Geometry check sheet. Reference: the model listing, model coordinates, mm. A direction names the side the tool comes from. Give positions to 0.01 mm unless a question says otherwise; leave off trailing zeros. Write each loop counter-clockwise with the first axis right and the second up, starting at its lowest first coordinate (ties: lowest second). Pieces come first, ordered by that corner, then holes. Notation, with made-up numbers: (-35.5, -11) -> (-4.5, -11) arc R17 ccw to (-4.5, 6) -> close; hole circle Ø5 at (33.5, 46.25). An arc over 180 degrees is marked (long way). One line per item, written item: value.
from build123d import *

# Parameters (mm, degrees)
BOSS_EXTRUDE1_DEPTH          = 3.175
SKETCH2_W                    = 2.75
SKETCH2_H                    = 2.5
SKETCH2_H_2                  = 4
SKETCH2_W_2                  = 1.125
SKETCH2_H_3                  = 7.5
CUT_EXTRUDE1_DEPTH           = 291.017379867
CIRPATTERN1_COUNT            = 4
F_3_0_3_DIAMETER_HOLE1_D     = 3
F_8_0_8_DIAMETER_HOLE1_D     = 8
F_8_0_8_DIAMETER_HOLE1_DEPTH = 6.35


with BuildPart() as part:
    # Sketch1 → Boss-Extrude1 (new, symmetric)
    with BuildSketch(Plane(origin=(0, 0, 0), x_dir=(1, 0, 0), z_dir=(0, 1, 0))):
        with BuildLine():
            Line((88.388347648, 98.994949366), (64.667874078, 75.274475795))
            ThreePointArc((64.667874078, 75.274475795), (-70.171862751, 70.171862751), (-75.274475795, -64.667874078))
            Line((-75.274475795, -64.667874078), (-98.994949366, -88.388347648))
            Line((-98.994949366, -88.388347648), (17.67766953, -205.060966544))
            Line((17.67766953, -205.060966544), (205.060966544, -17.67766953))
            Line((205.060966544, -17.67766953), (88.388347648, 98.994949366))
        make_face()
        with BuildLine():
            ThreePointArc((-64.667874078, -75.274475795), (0, -99.238), (64.667874078, -75.274475795))
            Line((64.667874078, -75.274475795), (95.45941546, -106.066017178))
            Line((95.45941546, -106.066017178), (17.67766953, -183.847763109))
            Line((17.67766953, -183.847763109), (-77.781745931, -88.388347648))
            Line((-77.781745931, -88.388347648), (-64.667874078, -75.274475795))
        make_face(mode=Mode.SUBTRACT)
        with BuildLine():
            ThreePointArc((75.274475795, -64.667874078), (99.238, 0), (75.274475795, 64.667874078))
            Line((75.274475795, 64.667874078), (88.388347648, 77.781745931))
            Line((88.388347648, 77.781745931), (183.847763109, -17.67766953))
            Line((183.847763109, -17.67766953), (106.066017178, -95.45941546))
            Line((106.066017178, -95.45941546), (75.274475795, -64.667874078))
        make_face(mode=Mode.SUBTRACT)
        with BuildLine():
            Line((-7.5, -7.5), (-7.5, -83.903460262))
            ThreePointArc((-7.5, -83.903460262), (-59.565261034, -59.565261034), (-83.903460262, -7.5))
            Line((-83.903460262, -7.5), (-7.5, -7.5))
        make_face(mode=Mode.SUBTRACT)
        with BuildLine():
            ThreePointArc((83.903460262, -7.5), (59.565261034, -59.565261034), (7.5, -83.903460262))
            Line((7.5, -83.903460262), (7.5, -7.5))
            Line((7.5, -7.5), (83.903460262, -7.5))
        make_face(mode=Mode.SUBTRACT)
        with BuildLine():
            Line((-7.5, 7.5), (-83.903460262, 7.5))
            ThreePointArc((-83.903460262, 7.5), (-59.565261034, 59.565261034), (-7.5, 83.903460262))
            Line((-7.5, 83.903460262), (-7.5, 7.5))
        make_face(mode=Mode.SUBTRACT)
        with BuildLine():
            ThreePointArc((7.5, 83.903460262), (59.565261034, 59.565261034), (83.903460262, 7.5))
            Line((83.903460262, 7.5), (7.5, 7.5))
            Line((7.5, 7.5), (7.5, 83.903460262))
        make_face(mode=Mode.SUBTRACT)
    extrude(amount=BOSS_EXTRUDE1_DEPTH, both=True)

    # Sketch2 → Cut-Extrude1 (cut, symmetric)
    with BuildSketch(Plane(origin=(0, 0, 0), x_dir=(1, 0, 0), z_dir=(0, 1, 0))):
        with Locations((0, 86.488)):
            Rectangle(SKETCH2_W, SKETCH2_H)
        with Locations((0, 89.738)):
            Rectangle(SKETCH2_W, SKETCH2_H_2)
        with Locations((1.9375, 89.738)):
            Rectangle(SKETCH2_W_2, SKETCH2_H_2)
        with Locations((0, 95.488)):
            Rectangle(SKETCH2_W, SKETCH2_H_3)
        with Locations((-1.9375, 89.738)):
            Rectangle(SKETCH2_W_2, SKETCH2_H_2)
    cut_extrude1 = extrude(amount=CUT_EXTRUDE1_DEPTH, both=True, mode=Mode.SUBTRACT)

    # CirPattern1: Cut-Extrude1 ×4 about axis
    cirpattern1_axis = Axis((0, 0, 0), (0, 1, 0))
    for i in range(1, CIRPATTERN1_COUNT):
        add(cut_extrude1.rotate(cirpattern1_axis, i * 360 / CIRPATTERN1_COUNT), mode=Mode.SUBTRACT)

    # Ø3.0 (3) Diameter Hole1 (through all)
    with Locations(Plane(origin=(0, 3.175, 0), x_dir=(1, 0, 0), z_dir=(0, 1, 0))):
        with Locations((-64.868561892, -64.868561892), (0, 0), (-64.868561892, 64.868561892), (64.868561892, 64.868561892), (64.868561892, -64.868561892)):
            Hole(F_3_0_3_DIAMETER_HOLE1_D / 2)

    # Ø8.0 (8) Diameter Hole1
    with Locations(Plane(origin=(0, 3.175, 0), x_dir=(1, 0, 0), z_dir=(0, 1, 0))):
        with Locations((0, 0)):
            Hole(F_8_0_8_DIAMETER_HOLE1_D / 2, depth=F_8_0_8_DIAMETER_HOLE1_DEPTH)


solid = part.part
1) Depth check by flat-ended pin: pin 1 Ø2 at (y, z) = (2.5, 69.5) entering from +X; pin 2 Ø2.5 at (x, z) = (64.87, 64.87) entering from -Y; pin 3 Ø1.5 at (x, y) = (-67.5, -2) entering from +Z; pin 4 Ø1 at (x, y) = (59.5, -2) entering from +Z. Enter the tip coordinate at first touch or a pass-through.
Verdict:
pin 1: x = 154.24
pin 2: through
pin 3: z = 120.63
pin 4: z = 163.74
2) Sectioned sample at A-A on x = -15. Record the cut outline in (y, z) (3 decimals).
Verdict:
outline: (-3.175, -98.098) -> (3.175, -98.098) -> (3.175, -82.892) -> (-3.175, -82.892) -> close; (-3.175, -7.5) -> (3.175, -7.5) -> (3.175, 7.5) -> (-3.175, 7.5) -> close; (-3.175, 82.892) -> (3.175, 82.892) -> (3.175, 98.098) -> (-3.175, 98.098) -> close; (-3.175, 151.17) -> (3.175, 151.17) -> (3.175, 172.383) -> (-3.175, 172.383) -> close
3) Sectioned sample at B-B on z = -15. Record the cut outline in (x, y) (3 decimals), plus the area to 3 significant figures.
Verdict:
outline: (-98.098, -3.175) -> (-82.892, -3.175) -> (-82.892, 3.175) -> (-98.098, 3.175) -> close; (-7.5, -3.175) -> (7.5, -3.175) -> (7.5, 3.175) -> (-7.5, 3.175) -> close; (82.892, -3.175) -> (98.098, -3.175) -> (98.098, 3.175) -> (82.892, 3.175) -> close; (151.17, -3.175) -> (172.383, -3.175) -> (172.383, 3.175) -> (151.17, 3.175) -> close
area: 423 mm^2
4) Mould release check, pull along X, two halves, no side actions. Record for faces 1 (the cylindrical face through (92.64, 0.04, 35.58)), 2 (the cylindrical face through (34.674, 0.044, 92.983)), 3 (the cylindrical face through (-92.983, 0.044, 34.674)), 4 (the flat face through (30, -3.175, 7)): released by +X, released by -X, zero draft, split by the parting line, or undercut.
Verdict:
face 1: undercut
face 2: undercut
face 3: released by -X
face 4: zero draft
5) Tool access check on faces 5 (the flat face through (135.45, 0.04, -30.72)), 6 (the flat face through (110.06, 0.04, 112.68)), 7 (the cylindrical face through (35.58, 0.04, -92.64)). Record the directions out of +Z, -Z, +X, -X, +Y, -Y that give a thin tool (end or side, any length) a straight path to the whole face; none if there is none.
Verdict:
face 5: +Y, -Y
face 6: +Z, +X, +Y, -Y
face 7: -Z, +Y, -Y
6) Scan lines: probe 1 along X at (y, z) = (2.5, 27.5); probe 2 along Z at (x, y) = (46, 0.75); probe 3 along Z at (x, y) = (-70.5, 1.75). Record each from-to range of solid material in increasing order.
Verdict:
probe 1: -95.35 to -79.62, -7.5 to 7.5, 79.62 to 95.35, 174.03 to 195.24
probe 2: -87.93 to -70.57, -7.5 to 7.5, 70.57 to 87.93, 155.53 to 176.74
probe 3: -69.84 to -46.11, -7.5 to 7.5, 46.11 to 81.11, 95.67 to 116.88
7) Sectioned sample at D-D on y = 0.5. Give the number of separate pieces and of enclosed holes in the cut face, plus the area to 3 significant figures.
Verdict:
separate pieces: 1
enclosed holes: 11
area: 22,900 mm^2
8) Sectioned sample at C-C on z = 140.5. Record the cut outline in (x, y) (3 decimals).
Verdict:
outline: (-46.883, -3.175) -> (-25.67, -3.175) -> (-25.67, 3.175) -> (-46.883, 3.175) -> close; (61.025, -3.175) -> (82.239, -3.175) -> (82.239, 3.175) -> (61.025, 3.175) -> close
